Check sheet for the modelled part. Datum: model origin and axes. Units: mm. Face numbers are marked on the shaded views. A direction names the side the tool comes from. Give positions to 0.01 mm unless a question says otherwise; leave off trailing zeros. Order: outer loops, then holes, each group sorted by start corner. A loop starts at its lowest first (then second) coordinate and runs counter-clockwise, first axis right, second up. Notation, with made-up numbers: (-24, -9) -> (27, -9) arc R18 cw to (27, 18) -> close; hole circle Ø8 at (16, -18.5). An arc over 180 degrees is marked (long way). One line per question, with ' | ' between items.
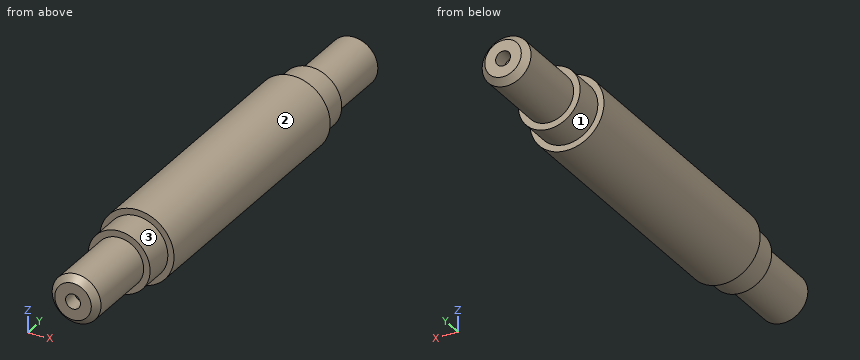
```python
from build123d import *

# Parameters (mm, degrees)
SKETCH4_R           = 3.95
SKETCH4_R_2         = 1.2
BOSS_EXTRUDE2_DEPTH = 18
CUT_EXTRUDE2_START  = 15.5
SKETCH4_3_R         = 1.2
CUT_EXTRUDE2_DEPTH  = 2.5
SKETCH4_4_R         = 5
SKETCH4_4_R_2       = 3.95
BOSS_EXTRUDE3_DEPTH = 5
BOSS_EXTRUDE4_START = -44
SKETCH4_5_R         = 6
SKETCH4_5_R_2       = 5
SKETCH4_5_R_3       = 3.95
SKETCH4_5_R_4       = 1.2
BOSS_EXTRUDE4_DEPTH = 44
BOSS_EXTRUDE8_START = -49
SKETCH4_10_R        = 5
SKETCH4_10_R_2      = 3.95
SKETCH4_10_R_3      = 1.2
BOSS_EXTRUDE8_DEPTH = 49
BOSS_EXTRUDE9_START = -62
SKETCH4_11_R        = 3.95
SKETCH4_11_R_2      = 1.2
BOSS_EXTRUDE9_DEPTH = 62
CUT_EXTRUDE3_START  = -59.5
SKETCH4_13_R        = 1.2
CUT_EXTRUDE3_DEPTH  = 4.077951389
CHAMFER3_SIZE       = 1


with BuildPart() as part:
    # Sketch4 → Boss-Extrude2 (new body)
    # profile 1 of 2: a face of its own
    with BuildSketch(Plane(origin=(0, 0, 0), x_dir=(1, 0, 0), z_dir=(0, 1, 0))):
        with Locations(Location((0, 0, 0), (0, 0, 270))):
            Circle(SKETCH4_R)
        Circle(SKETCH4_R_2, mode=Mode.SUBTRACT)
    # profile 2 of 2: a face of its own
    with BuildSketch(Plane(origin=(0, 0, 0), x_dir=(1, 0, 0), z_dir=(0, 1, 0))):
        Circle(SKETCH4_R_2)
    extrude(amount=BOSS_EXTRUDE2_DEPTH)

    # Sketch4_3 → Cut-Extrude2 (cut)
    with BuildSketch(Plane(origin=(0, 0, 0), x_dir=(1, 0, 0), z_dir=(0, 1, 0)).offset(CUT_EXTRUDE2_START)):
        with Locations(Location((0, 0, 0), (0, 0, 270))):
            Circle(SKETCH4_3_R)
    extrude(amount=CUT_EXTRUDE2_DEPTH, mode=Mode.SUBTRACT)

    # Sketch4_4 → Boss-Extrude3 (add)
    with BuildSketch(Plane(origin=(0, 0, 0), x_dir=(1, 0, 0), z_dir=(0, 1, 0))):
        with Locations(Location((0, 0, 0), (0, 0, 270))):
            Circle(SKETCH4_4_R)
        with Locations(Location((0, 0, 0), (0, 0, 270))):
            Circle(SKETCH4_4_R_2, mode=Mode.SUBTRACT)
    extrude(amount=BOSS_EXTRUDE3_DEPTH)

    # Sketch4_5 → Boss-Extrude4 (add)
    # profile 1 of 4: a face of its own
    with BuildSketch(Plane(origin=(0, 0, 0), x_dir=(1, 0, 0), z_dir=(0, 1, 0)).offset(BOSS_EXTRUDE4_START)):
        with Locations(Location((0, 0, 0), (0, 0, 270))):
            Circle(SKETCH4_5_R)
        with Locations(Location((0, 0, 0), (0, 0, 270))):
            Circle(SKETCH4_5_R_2, mode=Mode.SUBTRACT)
    # profile 2 of 4: a face of its own
    with BuildSketch(Plane(origin=(0, 0, 0), x_dir=(1, 0, 0), z_dir=(0, 1, 0)).offset(BOSS_EXTRUDE4_START)):
        with Locations(Location((0, 0, 0), (0, 0, 270))):
            Circle(SKETCH4_5_R_2)
        with Locations(Location((0, 0, 0), (0, 0, 270))):
            Circle(SKETCH4_5_R_3, mode=Mode.SUBTRACT)
    # profile 3 of 4: a face of its own
    with BuildSketch(Plane(origin=(0, 0, 0), x_dir=(1, 0, 0), z_dir=(0, 1, 0)).offset(BOSS_EXTRUDE4_START)):
        with Locations(Location((0, 0, 0), (0, 0, 270))):
            Circle(SKETCH4_5_R_3)
        with Locations(Location((0, 0, 0), (0, 0, 270))):
            Circle(SKETCH4_5_R_4, mode=Mode.SUBTRACT)
    # profile 4 of 4: a face of its own
    with BuildSketch(Plane(origin=(0, 0, 0), x_dir=(1, 0, 0), z_dir=(0, 1, 0)).offset(BOSS_EXTRUDE4_START)):
        with Locations(Location((0, 0, 0), (0, 0, 270))):
            Circle(SKETCH4_5_R_4)
    extrude(amount=BOSS_EXTRUDE4_DEPTH)

    # Sketch4_10 → Boss-Extrude8 (add)
    # profile 1 of 3: a face of its own
    with BuildSketch(Plane(origin=(0, 0, 0), x_dir=(1, 0, 0), z_dir=(0, 1, 0)).offset(BOSS_EXTRUDE8_START)):
        with Locations(Location((0, 0, 0), (0, 0, 270))):
            Circle(SKETCH4_10_R)
        with Locations(Location((0, 0, 0), (0, 0, 270))):
            Circle(SKETCH4_10_R_2, mode=Mode.SUBTRACT)
    # profile 2 of 3: a face of its own
    with BuildSketch(Plane(origin=(0, 0, 0), x_dir=(1, 0, 0), z_dir=(0, 1, 0)).offset(BOSS_EXTRUDE8_START)):
        with Locations(Location((0, 0, 0), (0, 0, 270))):
            Circle(SKETCH4_10_R_2)
        with Locations(Location((0, 0, 0), (0, 0, 270))):
            Circle(SKETCH4_10_R_3, mode=Mode.SUBTRACT)
    # profile 3 of 3: a face of its own
    with BuildSketch(Plane(origin=(0, 0, 0), x_dir=(1, 0, 0), z_dir=(0, 1, 0)).offset(BOSS_EXTRUDE8_START)):
        with Locations(Location((0, 0, 0), (0, 0, 270))):
            Circle(SKETCH4_10_R_3)
    extrude(amount=BOSS_EXTRUDE8_DEPTH)

    # Sketch4_11 → Boss-Extrude9 (add)
    # profile 1 of 2: a face of its own
    with BuildSketch(Plane(origin=(0, 0, 0), x_dir=(1, 0, 0), z_dir=(0, 1, 0)).offset(BOSS_EXTRUDE9_START)):
        with Locations(Location((0, 0, 0), (0, 0, 270))):
            Circle(SKETCH4_11_R)
        with Locations(Location((0, 0, 0), (0, 0, 270))):
            Circle(SKETCH4_11_R_2, mode=Mode.SUBTRACT)
    # profile 2 of 2: a face of its own
    with BuildSketch(Plane(origin=(0, 0, 0), x_dir=(1, 0, 0), z_dir=(0, 1, 0)).offset(BOSS_EXTRUDE9_START)):
        with Locations(Location((0, 0, 0), (0, 0, 270))):
            Circle(SKETCH4_11_R_2)
    extrude(amount=BOSS_EXTRUDE9_DEPTH)

    # Sketch4_13 → Cut-Extrude3 (cut, through all)
    with BuildSketch(Plane(origin=(0, 0, 0), x_dir=(1, 0, 0), z_dir=(0, 1, 0)).offset(CUT_EXTRUDE3_START)):
        with Locations(Location((0, 0, 0), (0, 0, 270))):
            Circle(SKETCH4_13_R)
    extrude(amount=-CUT_EXTRUDE3_DEPTH, mode=Mode.SUBTRACT)

    # Chamfer3
    chamfer3_edges = [part.edges().sort_by_distance(p)[0] for p in [
        (0, -62, -3.95),
        (0, 18, -3.95),
    ]]
    chamfer(chamfer3_edges, length=CHAMFER3_SIZE)


solid = part.part
```
Q1. Access from +Z, -Z, +X, -X, +Y, -Y to the whole of each face (thin tool, end or side, straight path). Record for the marked faces 1, 2 and 3.
Result sheet:
face 1: +Y | face 2: +Y, -Y | face 3: -Y
Q2. Section check C-C (y = -8). Enter the section's corners in (x, z).
Result sheet:
outline: circle Ø12 at (0, 0)
Q3. Depth check by flat-ended pin: pin 1 Ø1.2 at (x, z) = (-0.5, -0.5) entering from -Y; pin 2 Ø6 at (x, y) = (2.5, -46.5) entering from -Z; pin 3 Ø3 at (y, z) = (-52, 4) entering from -X; pin 4 Ø1.9 at (x, z) = (0, 0) entering from -Y. Enter the tip coordinate at first touch or a pass-through.
Result sheet:
pin 1: stops at y = -62 | pin 2: stops at z = -5.94 | pin 3: stops at x = -3.06 | pin 4: stops at y = -59.5
Q4. Thickness scan on line 1 (X direction, y = 16.6, z = 0); line 2 (Y direction, x = 4.75, z = 0); line 3 (Z direction, x = -0.25, y = 10). Record the ranges inside material, lowest first.
Result sheet:
line 1: x = -3.95 to -1.2, 1.2 to 3.95 | line 2: y = -49 to 5 | line 3: z = -3.94 to 3.94
